Could you check a few things on this model? Use its own coordinates, in mm. A direction names the side the tool comes from. Coordinates: 2 decimals unless noted, no trailing zeros. Loops run counter-clockwise (first coordinate to the right, second up) from the corner with the lowest first, then second, coordinate; pieces in that order, holes last. Notation, with made-up numbers: (78.25, -11.75) -> (119.25, -11.75) arc R24 ccw to (119.25, 4.25) -> close; hole circle Ø8 at (-38.75, 26.5). An arc over 180 degrees is marked (long way). One line per question, with ' | ' between items. Start each with the question number.
(1) Suppose I cut it at C-C (x = 41). Please give me the cut outline in (y, z).
(2) Which directions (+Z, -Z, +X, -X, +Y, -Y) give clear straight access to the entire face, cutting with the end or side of a thin tool? Please do faces 5 (the face through (-47.5, 6, 14)), 6 (the face through (-1, 5, -39.706)).
(3) Suppose I cut it at B-B (z = -4). Please give me the cut outline in (x, y).
(4) I'm going to push a flat-ended pin straight in: pin 1 Ø2 at (x, z) = (17, -26.5) entering from +Y. Where does the tip first touch, or does it pass through?
(5) Suppose I cut it at A-A (y = 7.5). Please give me the cut outline in (x, z).
(6) If we mould it in two halves opening along Z, with no side actions, what happens to faces 1 (the face through (-1, 5, 69.294)), 2 (the face through (-51.5, 5, 14)), 3 (the face through (-1, 2, 14)), 4 (the face through (47.5, 6, 16))? For each: pulls with the +Z half, pulls with the -Z half, needs draft (parallel to the pull), parting line crosses it, or undercut.
(7) If I drill on line 1 along Z through (x, y) = (8.5, 6.25); line 2 along X through (y, z) = (5, 34); line 3 along Y through (x, z) = (39.5, 9.5), over which ranges is the centre line in solid material (lowest first)?
```python
from build123d import *

# Parameters (mm, degrees)
SKETCH1_W           = 95
SKETCH1_H           = 101
BOSS_EXTRUDE1_DEPTH = 2
SKETCH2_W           = 103
SKETCH2_H           = 109
BOSS_EXTRUDE2_DEPTH = 7
CUT_EXTRUDE1_DEPTH  = 7
SKETCH4_W           = 103
SKETCH4_H           = 109
BOSS_EXTRUDE9_DEPTH = 2


with BuildPart() as part:
    # Sketch1 → Boss-Extrude1 (new body)
    with BuildSketch(Plane(origin=(0, 0, 0), x_dir=(1, 0, 0), z_dir=(0, 1, 0))):
        with Locations((0, -14.793667886)):
            Rectangle(SKETCH1_W, SKETCH1_H)
    extrude(amount=BOSS_EXTRUDE1_DEPTH)

    # Sketch2 → Boss-Extrude2 (add)
    with BuildSketch(Plane(origin=(0, 2, 0), x_dir=(1, 0, 0), z_dir=(0, 1, 0))):
        with Locations((0, -14.793667886)):
            Rectangle(SKETCH2_W, SKETCH2_H)
    extrude(amount=BOSS_EXTRUDE2_DEPTH)

    # Sketch3 → Cut-Extrude1 (cut)
    with BuildSketch(Plane(origin=(0, 9, 0), x_dir=(1, 0, 0), z_dir=(0, 1, 0))):
        Polygon((47.5, -65.060658177), (-47.5, 35.473322405), (-47.5, -65.293667886), (47.5, -65.293667886), align=None)
        Polygon((-47.5, 35.706332114), (-47.5, 35.473322405), (47.5, -65.060658177), (47.5, 35.706332114), align=None)
    extrude(amount=-CUT_EXTRUDE1_DEPTH, mode=Mode.SUBTRACT)

    # Sketch4 → Boss-Extrude9 (add, through all)
    with BuildSketch(Plane.XZ.offset(-2)):
        with Locations((0, 14.793667886)):
            Rectangle(SKETCH4_W, SKETCH4_H)
    extrude(amount=BOSS_EXTRUDE9_DEPTH)


solid = part.part
```
Checks:
1) outline: (0, -39.71) -> (9, -39.71) -> (9, -35.71) -> (2, -35.71) -> (2, 65.29) -> (9, 65.29) -> (9, 69.29) -> (0, 69.29) -> close
2) face 5: +Y | face 6: -Z, +X, -X, +Y, -Y
3) outline: (-51.5, 0) -> (51.5, 0) -> (51.5, 9) -> (47.5, 9) -> (47.5, 2) -> (-47.5, 2) -> (-47.5, 9) -> (-51.5, 9) -> close
4) pin 1: stops at y = 2
5) outline: (-51.5, -39.71) -> (51.5, -39.71) -> (51.5, 69.29) -> (-51.5, 69.29) -> close; hole (-47.5, -35.71) -> (47.5, -35.71) -> (47.5, 65.29) -> (-47.5, 65.29) -> close
6) face 1: pulls with the +Z half | face 2: needs draft | face 3: undercut | face 4: undercut
7) line 1: z = -39.71 to -35.71, 65.29 to 69.29 | line 2: x = -51.5 to -47.5, 47.5 to 51.5 | line 3: y = 0 to 2
